Here's how the part is built. I have some questions about the finished solid (model axes, mm). A direction names the side the tool comes from. Give positions to 0.01 mm unless a question says otherwise; leave off trailing zeros. Write each loop counter-clockwise with the first axis right and the second up, starting at its lowest first coordinate (ties: lowest second). Pieces come first, ordered by that corner, then holes. Notation, with made-up numbers: (52.25, 82.25) -> (76.25, 82.25) arc R21 cw to (76.25, 94.25) -> close; hole circle Ø5 at (-24, -31). An arc over 180 degrees is marked (long way). Use CSV: the item, a comma, the result in double quotes. Start each with the question number.
(1) Suppose I cut it at C-C on z = -1. List the corners of the cut face in (x, y) for me (3 decimals).
(2) Suppose I cut it at A-A on y = 2.25. List the corners of the cut face in (x, z) for me.
(3) Suppose I cut it at B-B on x = 3.75. List the corners of the cut face in (y, z) for me (3 decimals).
(4) For pin 1 Ø0.8 at (x, y) = (8.5, 2.5) entering from +Z; pin 2 Ø0.8 at (y, z) = (2, -5) entering from -X; pin 3 Ø0.5 at (y, z) = (2.5, -2.5) entering from -X; pin 4 Ø0.8 at (x, y) = (8, 2.5) entering from -Z, each with a flat end and sliding along its axis, tell me the tip position at first contact or that it passes through.
(5) Which directions (+Z, -Z, +X, -X, +Y, -Y) give clear straight access to the entire face, cutting with the end or side of a thin tool? Please do faces 1 (the flat face through (0.584, 2.4, -5)), 2 (the flat face through (8.2, 2.4, -6.794)), 3 (the flat face through (3.302, 2.4, -1.9)), 4 (the flat face through (3.302, 2.4, -8.2)).
(6) Suppose I cut it at D-D on x = 9.75. List the corners of the cut face in (y, z) for me (3 decimals).
(7) I need wall thicknesses on L1, parallel to X at y = 2.65, z = -4; L2, parallel to Z at x = 6.5, y = 2.6; L3, parallel to Y at x = 8.25, z = -7.25 (3 decimals). Which ranges of each line are inside material? Lowest first, please. Write a range as [from, to].
from build123d import *

# Parameters (mm, degrees)
SKETCH1_W           = 10.16
SKETCH1_H           = 10.16
BOSS_EXTRUDE1_DEPTH = 1.905
SKETCH2_W           = 3.556
SKETCH2_H           = 8.9916
BOSS_EXTRUDE4_DEPTH = 2.8702
SKETCH4_W           = 8.9916
SKETCH4_H           = 3.556
BOSS_EXTRUDE5_DEPTH = 2.8702


with BuildPart() as part:
    # Sketch1 → Boss-Extrude1 (new body)
    with BuildSketch(Plane(origin=(0, 0, 0), x_dir=(1, 0, 0), z_dir=(0, 1, 0))):
        with Locations((5.08, 5.08)):
            Rectangle(SKETCH1_W, SKETCH1_H)
    extrude(amount=BOSS_EXTRUDE1_DEPTH)

    # Sketch2 → Boss-Extrude4 (add)
    with BuildSketch(Plane(origin=(0, 0, 0), x_dir=(1, 0, 0), z_dir=(0, 1, 0))):
        with Locations((5.08, 5.08)):
            Rectangle(SKETCH2_W, SKETCH2_H)
    extrude(amount=BOSS_EXTRUDE4_DEPTH)

    # Sketch4 → Boss-Extrude5 (add)
    with BuildSketch(Plane(origin=(0, 0, 0), x_dir=(1, 0, 0), z_dir=(0, 1, 0))):
        with Locations((5.08, 5.0165)):
            Rectangle(SKETCH4_W, SKETCH4_H)
    extrude(amount=BOSS_EXTRUDE5_DEPTH)


solid = part.part
Geometry says:
1,outline,"(0, 0) -> (10.16, 0) -> (10.16, 1.905) -> (6.858, 1.905) -> (6.858, 2.87) -> (3.302, 2.87) -> (3.302, 1.905) -> (0, 1.905) -> close"
2,outline,"(0.58, -6.79) -> (3.3, -6.79) -> (3.3, -9.58) -> (6.86, -9.58) -> (6.86, -6.79) -> (9.58, -6.79) -> (9.58, -3.24) -> (6.86, -3.24) -> (6.86, -0.58) -> (3.3, -0.58) -> (3.3, -3.24) -> (0.58, -3.24) -> close"
3,outline,"(0, -10.16) -> (1.905, -10.16) -> (1.905, -9.576) -> (2.87, -9.576) -> (2.87, -0.584) -> (1.905, -0.584) -> (1.905, 0) -> (0, 0) -> close"
4,pin 1,"z = -3.24"
4,pin 2,"x = 0"
4,pin 3,"x = 3.3"
4,pin 4,"z = -6.79"
5,face 1,"+Z, -Z, -X, +Y"
5,face 2,"-Z, +X, +Y"
5,face 3,"+Z, -X, +Y"
5,face 4,"-Z, -X, +Y"
6,outline,"(0, -10.16) -> (1.905, -10.16) -> (1.905, 0) -> (0, 0) -> close"
7,L1,"[0.58, 9.58]"
7,L2,"[-9.58, -0.58]"
7,L3,"[0, 1.905]"
